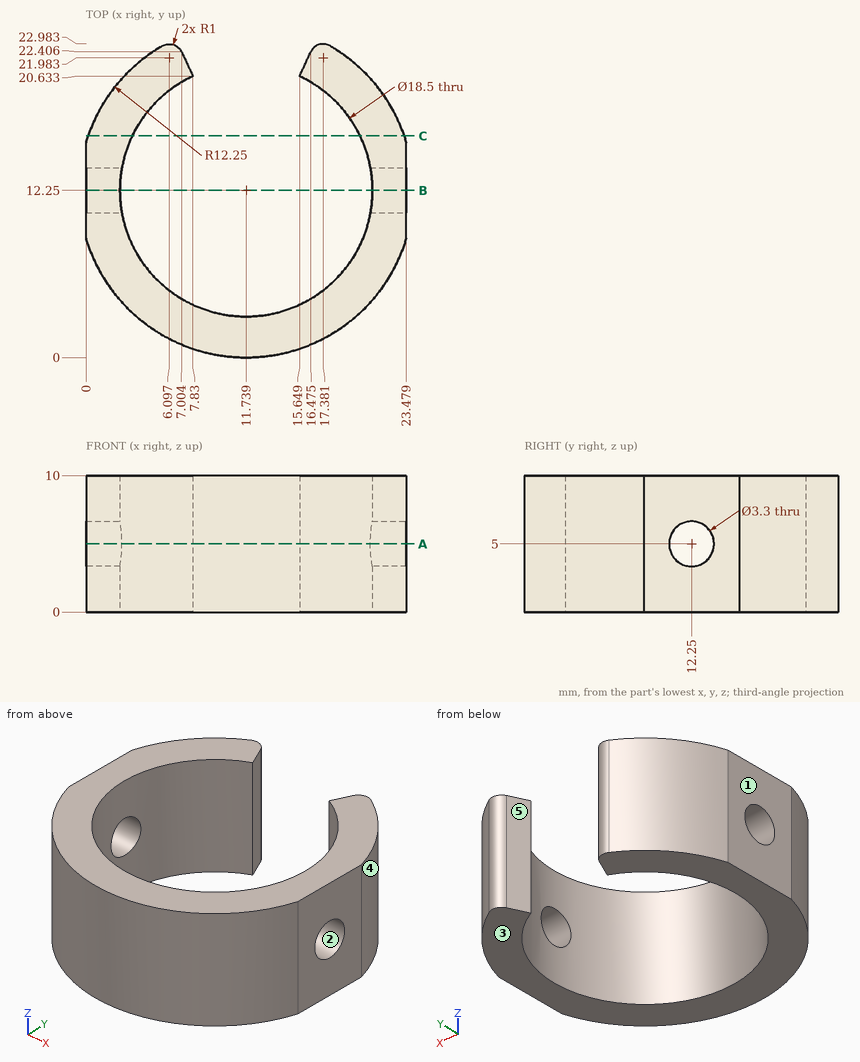
Job drawing, mm, ordinate dimensions from the low corner. One solid piece. A direction names the side the tool comes from. Give positions to 0.01 mm unless a question says otherwise; leave off trailing zeros. Write each loop counter-clockwise with the first axis right and the second up, starting at its lowest first coordinate (ties: lowest second). Pieces come first, ordered by that corner, then holes. Notation, with made-up numbers: (78.5, 70.25) - (123.5, 70.25) arc R27 ccw to (123.5, 89.25) - close; hole circle Ø5 at (-34.5, 30). An arc over 180 degrees is marked (long way). Answer as CSV lines item,"result".
1. Two-plate mould, pull along Z, no slides. Class the marked faces 1, 2 and 3: +Z half, -Z half, draft (parallel to the pull), parting line (faces both ways), or undercut.
Responses:
face 1,"draft"
face 2,"undercut"
face 3,"-Z half"
2. Band-saw the part on A-A (z = 5). Count the separate pieces of the cut face and the enclosed holes in it.
Responses:
separate pieces,"3"
enclosed holes,"0"
3. Band-saw the part on B-B (y = 12.25). Write the cut outline in (x, z).
Responses:
outline,"(0, 0) - (2.49, 0) - (2.49, 3.35) - (0, 3.35) - close; (0, 6.65) - (2.49, 6.65) - (2.49, 10) - (0, 10) - close; (20.99, 0) - (23.48, 0) - (23.48, 3.35) - (20.99, 3.35) - close; (20.99, 6.65) - (23.48, 6.65) - (23.48, 10) - (20.99, 10) - close"
4. Pin check, flat tips, straight feed: pin 1 (1.5 mm diameter, centred on y = 18, z = 3, fed in from -X); pin 2 (5 mm diameter, centred on x = 3, z = 1, fed in from -Y); pin 3 (2 mm diameter, centred on x = 3, z = 1.5, fed in from +Y) (1 decimal). Stop position of each tip, or through.
Responses:
pin 1,"stops at x = 0.56"
pin 2,"stops at y = 1.71"
pin 3,"stops at y = 21.7"
5. Band-saw the part on C-C (y = 16.25). Write the cut outline in (x, z).
Responses:
outline,"(0.16, 0) - (3.4, 0) - (3.4, 10) - (0.16, 10) - close; (20.08, 0) - (23.32, 0) - (23.32, 10) - (20.08, 10) - close"
6. Drill centre lines: L1, parallel to Z at x = 0.95, y = 12.25; L2, parallel to X at y = 12.25, z = 1; L3, parallel to X at y = 8.25, z = 7.5. Where is each one in solid material? Low to high. Write a range as [from, to].
Responses:
L1,"z = [0, 3.35], [6.65, 10]"
L2,"x = [0, 2.49], [20.99, 23.48]"
L3,"x = [0.16, 3.4], [20.08, 23.32]"
7. 3-axis set-ups, long thin cutter, end or side, ignore diameter. For the marked faces 4 and 5: which of +Z, -Z, +X, -X, +Y, -Y reach the whole face in a straight line?
Responses:
face 4,"+Z, -Z, +X, +Y"
face 5,"+Z, -Z, +Y"
